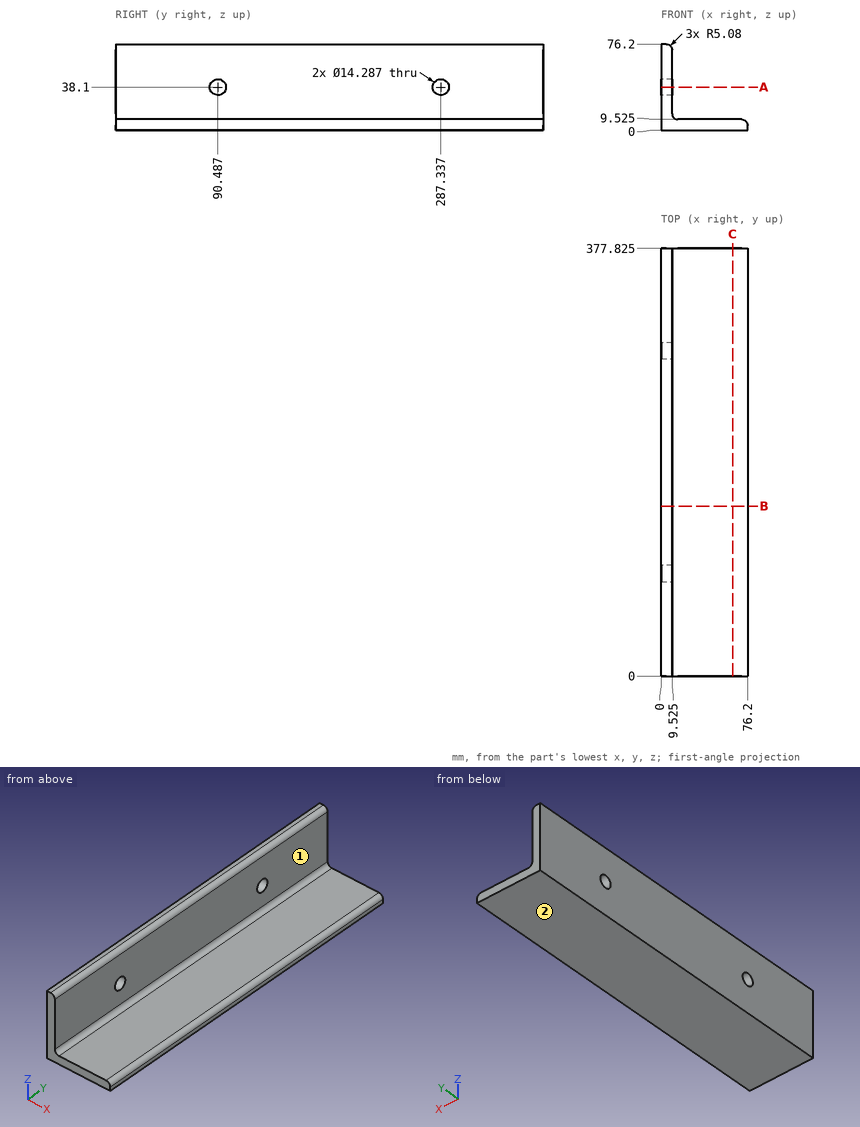
The drawing under review shows one solid part. Ordinate dimensions are in mm from its lowest x, y, z. A direction names the side the tool comes from. Round coordinates to 2 decimals unless told otherwise and drop trailing zeros. Loops run counter-clockwise (first coordinate to the right, second up) from the corner with the lowest first, then second, coordinate; pieces in that order, holes last.
Item 1: For the marked faces 1 and 2, list the 3-axis set-ups (+Z, -Z, +X, -X, +Y, -Y) from which the entire face can be reached by the end or side of a thin tool; tool diameter is ignored.
Determined:
face 1: +Z, +X, +Y, -Y
face 2: -Z, +X, -X, +Y, -Y
Item 2: Take a section at A-A (z = 38.1). Write out the cut boundary in (x, y) (1 decimal), then the cut area to 3 significant figures.
Determined:
outline: (0, 0) - (9.5, 0) - (9.5, 83.3) - (0, 83.3) - close; (0, 97.6) - (9.5, 97.6) - (9.5, 280.2) - (0, 280.2) - close; (0, 294.5) - (9.5, 294.5) - (9.5, 377.8) - (0, 377.8) - close
area: 3,330 mm2
Item 3: Clearance check with flat-ended pins moving along their axes: pin 1 Ø8 at (x, y) = (32.5, 308.5) entering from +Z (1 decimal); pin 2 Ø17 at (y, z) = (173, 41.5) entering from +X (1 decimal). State where each tip first meets the part, or that it passes through.
Determined:
pin 1: stops at z = 9.5
pin 2: stops at x = 9.5
Item 4: For line 1 (Y direction, x = 3, z = 38) (1 decimal); line 2 (X direction, y = 236.5, z = 26) (1 decimal), list the stretches that pass through material, from the lowest coordinate up.
Determined:
line 1: y = 0 to 83.3, 97.6 to 280.2, 294.5 to 377.8
line 2: x = 0 to 9.5
Item 5: Take a section at C-C (x = 63). Write out the cut boundary in (y, z) (1 decimal).
Determined:
outline: (0, 0) - (377.8, 0) - (377.8, 9.5) - (0, 9.5) - close
Item 6: Take a section at B-B (y = 150). Write out the cut boundary in (x, z) (1 decimal), then the cut area to 3 significant figures.
Determined:
outline: (0, 0) - (76.2, 0) - (76.2, 4.4) arc R5.1 ccw to (71.1, 9.5) - (14.6, 9.5) arc R5.1 cw to (9.5, 14.6) - (9.5, 71.1) arc R5.1 ccw to (4.4, 76.2) - (0, 76.2) - close
area: 1,360 mm2
